Geometry: final body of the model. Coordinates: model frame, mm. A direction names the side the tool comes from. Coordinates: 2 decimals unless noted, no trailing zeros. Order: outer loops, then holes, each group sorted by start corner. A loop starts at its lowest first (then second) coordinate and runs counter-clockwise, first axis right, second up. Notation, with made-up numbers: (-39, -20) -> (12, -20) arc R14 ccw to (12, -5) -> close; hole circle Ø10 at (-20, 63). An arc over 180 degrees is marked (long way). Use one line per item in the form item = value.
```python
from build123d import *

# Parameters (mm, degrees)
SKETCH1_W                                       = 43.18
SKETCH1_H                                       = 1346.2
BOSS_EXTRUDE1_DEPTH                             = 33.3248
SKETCH9_W                                       = 33.3375
SKETCH9_H                                       = 33.121582444
CUT_EXTRUDE1_DEPTH                              = 1348.304529308
CSK_FOR_10_FLAT_HEAD_MACHINE_SCREW3_D           = 5.1054
CSK_FOR_10_FLAT_HEAD_MACHINE_SCREW3_DEPTH       = 76.2
CSK_FOR_10_FLAT_HEAD_MACHINE_SCREW3_CSINK_D     = 10.2206044
CSK_FOR_10_FLAT_HEAD_MACHINE_SCREW3_CSINK_ANGLE = 82
CSK_FOR_10_FLAT_HEAD_MACHINE_SCREW3_TIP         = 1.533816902


with BuildPart() as part:
    # Sketch1 → Boss-Extrude1 (new body)
    with BuildSketch(Plane.XY):
        with Locations((-21.59, -548.180033686)):
            Rectangle(SKETCH1_W, SKETCH1_H)
    extrude(amount=BOSS_EXTRUDE1_DEPTH)

    # Sketch9 → Cut-Extrude1 (cut, through all)
    with BuildSketch(Plane(origin=(0, 124.919966314, 0), x_dir=(1, 0, 0), z_dir=(0, 1, 0))):
        with Locations((-21.81225, -8.826508778)):
            Rectangle(SKETCH9_W, SKETCH9_H)
    extrude(amount=-CUT_EXTRUDE1_DEPTH, mode=Mode.SUBTRACT)

    # CSK for #10 Flat Head Machine Screw3
    with Locations(Plane(origin=(0, 0, 25.3873), x_dir=(-1, 0, 0), z_dir=(0, 0, -1))):
        with Locations((21.59, -1183.180033686), (21.59, -1056.180033686), (21.59, -929.180033686), (21.59, -802.180033686), (21.59, -675.180033686), (21.59, -548.180033686), (21.59, -421.180033686), (21.59, -294.180033686), (21.59, -167.180033686), (21.59, -40.180033686), (21.59, 86.819966314)):
            CounterSinkHole(CSK_FOR_10_FLAT_HEAD_MACHINE_SCREW3_D / 2, CSK_FOR_10_FLAT_HEAD_MACHINE_SCREW3_CSINK_D / 2, depth=CSK_FOR_10_FLAT_HEAD_MACHINE_SCREW3_DEPTH, counter_sink_angle=CSK_FOR_10_FLAT_HEAD_MACHINE_SCREW3_CSINK_ANGLE)
            with Locations((0, 0, -(CSK_FOR_10_FLAT_HEAD_MACHINE_SCREW3_DEPTH + CSK_FOR_10_FLAT_HEAD_MACHINE_SCREW3_TIP / 2))):  # 118° drill point
                Cone(0, CSK_FOR_10_FLAT_HEAD_MACHINE_SCREW3_D / 2, CSK_FOR_10_FLAT_HEAD_MACHINE_SCREW3_TIP, mode=Mode.SUBTRACT)


solid = part.part
```
1) Section B-B, the plane y = -214.5. Output: boundary loops of the cut face in (x, z).
Results found:
outline = (-43.18, 0) -> (-38.48, 0) -> (-38.48, 25.39) -> (-5.14, 25.39) -> (-5.14, 0) -> (0, 0) -> (0, 33.32) -> (-43.18, 33.32) -> close
2) Contact query for flat-ended pins moving along their axis: P1, Ø4.5, axis at x = -21.59, y = -40.18, coming from the -Z side; P2, Ø12, axis at x = -12.5, y = -33, coming from the -Z side; P3, Ø6.5, axis at x = -21.59, y = 86.82, coming from the -Z side. Output: stop coordinate, or through.
Results found:
P1 = through
P2 = 25.39
P3 = 27.53
3) Material intervals for probe 1 along X at (y, z) = (-950, 18); probe 2 along Z at (x, y) = (-24.5, -851.5); probe 3 along Z at (x, y) = (-25, -802), sorted ascending. Write a range as from..to.
Results found:
probe_1 = -43.18..-38.48, -5.14..0
probe_2 = 25.39..33.32
probe_3 = 27.34..33.32
4) Section A-A, the plane z = 18. Output: boundary loops of the cut face in (x, y).
Results found:
outline = (-43.18, -1221.28) -> (-38.48, -1221.28) -> (-38.48, 124.92) -> (-43.18, 124.92) -> close; (-5.14, -1221.28) -> (0, -1221.28) -> (0, 124.92) -> (-5.14, 124.92) -> close
5) Access query for faces 1 (the flat face through (-22, -539, 25.387)), 2 (the flat face through (-22, -539, 33.325)). Directions: +Z, -Z, +X, -X, +Y, -Y. A direction counts if a zero-diameter tool reaches every point of the face in a straight line with its end or side. Return the directions, or none.
Results found:
face_1 = -Z, +Y, -Y
face_2 = +Z, +X, -X, +Y, -Y
6) Pull-direction query (X, two-part tool) for faces 3 (the flat face through (-43.18, -558, 16)), 4 (the flat face through (-22, -1221.28, 28)), 5 (the flat face through (-5.143, -539, 13)); classes: released by +X, released by -X, zero draft, split by the parting line, or undercut.
Results found:
face_3 = released by -X
face_4 = zero draft
face_5 = undercut
